```python
from build123d import *

# Parameters (mm, degrees)
PAD_DEPTH       = 5
PAD001_DEPTH    = 30
POCKET_DEPTH    = 162.001
POCKET001_DEPTH = 5
PAD002_DEPTH    = 5
POCKET002_DEPTH = 5.001
SKETCH007_W     = 22.303925
SKETCH007_H     = 15.153027
SKETCH007_W_2   = 15.272888
SKETCH007_H_2   = 13.786167
POCKET003_DEPTH = 3
SKETCH008_W     = 25.606406
SKETCH008_H     = 16.851532
SKETCH008_W_2   = 36.655319
SKETCH008_H_2   = 18.371552
POCKET004_DEPTH = 3
SKETCH009_R     = 1.5
POCKET005_DEPTH = 5
SKETCH010_R     = 3.6
SKETCH010_R_2   = 12.75
POCKET006_DEPTH = 5.001
SKETCH011_W     = 5.6250572961
SKETCH011_H     = 4
POCKET007_DEPTH = 5.001
SKETCH012_R     = 15
POCKET008_DEPTH = 3
SKETCH013_R     = 6.1
POCKET009_DEPTH = 1
SKETCH_R        = 1.4
POCKET010_DEPTH = 3.5
POCKET011_DEPTH = 0.2
SKETCH016_W     = 10
SKETCH016_H     = 12
POCKET013_DEPTH = 2.5
SKETCH018_W     = 7.2
SKETCH018_H     = 7.2
POCKET015_DEPTH = 0.2
POCKET016_DEPTH = 3
CHAMFER_SIZE    = 2.2
CHAMFER001_SIZE = 2.9


with BuildPart() as part:
    # Sketch001 → Pad (new body)
    with BuildSketch(Plane.XY):
        with BuildLine():
            Line((0, 0), (162, 0))
            Line((162, 0), (162, 61))
            ThreePointArc((162, 61), (158.4852813742, 69.4852813742), (150, 73))
            Line((150, 73), (12, 73))
            ThreePointArc((12, 73), (3.5147186258, 69.4852813742), (0, 61))
            Line((0, 61), (0, 0))
        make_face()
    extrude(amount=PAD_DEPTH)

    # Sketch002 (on Face8 of Pad) → Pad001 (join)
    with BuildSketch(Plane.XY.offset(5)):
        Polygon((0, 0), (0, 43), (3, 43), (3, 3), (159, 3), (159, 43), (162, 43), (162, 0), align=None)
    extrude(amount=PAD001_DEPTH)

    # Sketch003 (on Face10 of Pad001) → Pocket (cut, through all)
    with BuildSketch(Plane.YZ.offset(162)):
        Polygon((43, 5), (32.4169947557, 8), (23.0748598999, 18), (3, 27), (3, 35), (43, 35), align=None)
    extrude(amount=-POCKET_DEPTH, mode=Mode.SUBTRACT)

    # Sketch004 (on Face5 of Pocket) → Pocket001 (cut)
    with BuildSketch(Plane.XZ):
        with BuildLine():
            Line((0, 27), (0, 61.0433678259))
            Line((0, 61.0433678259), (162, 61.0433678259))
            Line((162, 61.0433678259), (162, 27))
            ThreePointArc((162, 27), (81, 35), (0, 27))
        make_face()
    extrude(amount=-POCKET001_DEPTH, mode=Mode.SUBTRACT)

    # Sketch005 (on Face7 of Pocket001) → Pad002 (join)
    with BuildSketch(Plane.XY.offset(5)):
        with BuildLine():
            Line((162, 50), (169.5, 50))
            ThreePointArc((172, 47.5), (171.267766953, 49.267766953), (169.5, 50))
            Line((172, 47.5), (172, 40.5))
            ThreePointArc((169.5, 38), (171.267766953, 38.732233047), (172, 40.5))
            Line((169.5, 38), (162, 38))
            Line((162, 38), (162, 50))
        make_face()
        with BuildLine():
            Line((0, 50), (-7.5, 50))
            ThreePointArc((-7.5, 50), (-9.267766953, 49.267766953), (-10, 47.5))
            Line((-10, 47.5), (-10, 40.5))
            ThreePointArc((-10, 40.5), (-9.267766953, 38.732233047), (-7.5, 38))
            Line((-7.5, 38), (0, 38))
            Line((0, 38), (0, 50))
        make_face()
        with BuildLine():
            Line((20.5, 73), (40.5, 73))
            Line((40.5, 73), (40.5, 80))
            ThreePointArc((40.5, 80), (39.6213203436, 82.1213203436), (37.5, 83))
            Line((37.5, 83), (23.5, 83))
            ThreePointArc((23.5, 83), (21.3786796564, 82.1213203436), (20.5, 80))
            Line((20.5, 80), (20.5, 73))
        make_face()
        with BuildLine():
            Line((121.5, 73), (141.5, 73))
            Line((141.5, 73), (141.5, 80))
            ThreePointArc((141.5, 80), (140.6213203436, 82.1213203436), (138.5, 83))
            Line((138.5, 83), (124.5, 83))
            ThreePointArc((124.5, 83), (122.3786796564, 82.1213203436), (121.5, 80))
            Line((121.5, 80), (121.5, 73))
        make_face()
    extrude(amount=-PAD002_DEPTH)

    # Sketch006 (on Face56 of Pad002) → Pocket002 (cut, through all)
    with BuildSketch(Plane.XY.offset(5)):
        with BuildLine():
            ThreePointArc((26, 80.5), (23.5, 78), (26, 75.5))
            Line((26, 75.5), (35, 75.5))
            ThreePointArc((35, 75.5), (37.5, 78), (35, 80.5))
            Line((35, 80.5), (26, 80.5))
        make_face()
        with BuildLine():
            ThreePointArc((127, 80.5), (124.5, 78), (127, 75.5))
            Line((127, 75.5), (136, 75.5))
            ThreePointArc((136, 75.5), (138.5, 78), (136, 80.5))
            Line((136, 80.5), (127, 80.5))
        make_face()
        with BuildLine():
            ThreePointArc((-15.2672618866, 46), (-17.2672618866, 44), (-15.2672618866, 42))
            Line((-15.2672618866, 42), (-6, 42))
            ThreePointArc((-6, 42), (-4, 44), (-6, 46))
            Line((-6, 46), (-15.2672618866, 46))
        make_face()
        with BuildLine():
            ThreePointArc((180.8359560682, 42), (182.8359560682, 44), (180.8359560682, 46))
            Line((180.8359560682, 46), (168, 46))
            ThreePointArc((168, 46), (166, 44), (168, 42))
            Line((168, 42), (180.8359560682, 42))
        make_face()
    extrude(amount=-POCKET002_DEPTH, mode=Mode.SUBTRACT)

    # Sketch007 (on Face29 of Pocket002) → Pocket003 (cut)
    with BuildSketch(Plane.XY.offset(5)):
        with Locations((-11.1519625, 45.5765135)):
            Rectangle(SKETCH007_W, SKETCH007_H)
        with Locations((169.636444, 43.1069165)):
            Rectangle(SKETCH007_W_2, SKETCH007_H_2)
    extrude(amount=-POCKET003_DEPTH, mode=Mode.SUBTRACT)

    # Sketch008 (on Face4 of Pocket003) → Pocket004 (cut)
    with BuildSketch(Plane(origin=(0, 0, 0), x_dir=(1, 0, 0), z_dir=(0, 0, -1))):
        with Locations((27.696797, -81.425766)):
            Rectangle(SKETCH008_W, SKETCH008_H)
        with Locations((139.8276595, -82.185776)):
            Rectangle(SKETCH008_W_2, SKETCH008_H_2)
    extrude(amount=-POCKET004_DEPTH, mode=Mode.SUBTRACT)

    # Sketch009 (on Face29 of Pocket004) → Pocket005 (cut)
    with BuildSketch(Plane.XY.offset(5)):
        with Locations((138.5, 78)):
            Circle(SKETCH009_R)
        with Locations((23.5, 78)):
            Circle(SKETCH009_R)
    extrude(amount=-POCKET005_DEPTH, mode=Mode.SUBTRACT)

    # Sketch010 (on Face65 of Pocket005) → Pocket006 (cut, through all)
    with BuildSketch(Plane.XY.offset(5)):
        with Locations((68.4, 38)):
            Circle(SKETCH010_R)
        with Locations((31.0483132961, 45)):
            Circle(SKETCH010_R_2)
        Polygon((88.4, 55), (151, 55), (151, 16), (138.5, 16), (136.5000000003, 14), (102.9, 14), (100.9, 16), (88.4, 16), align=None)
    extrude(amount=-POCKET006_DEPTH, mode=Mode.SUBTRACT)

    # Sketch011 (on Face69 of Pocket006) → Pocket007 (cut, through all)
    with BuildSketch(Plane.XY.offset(5)):
        with Locations((42.985784648, 45)):
            Rectangle(SKETCH011_W, SKETCH011_H)
    extrude(amount=-POCKET007_DEPTH, mode=Mode.SUBTRACT)

    # Sketch012 (on Face42 of Pocket007) → Pocket008 (cut)
    with BuildSketch(Plane.XY.offset(5)):
        with Locations((31.0483132961, 45)):
            Circle(SKETCH012_R)
    extrude(amount=-POCKET008_DEPTH, mode=Mode.SUBTRACT)

    # Sketch013 (on Face72 of Pocket008) → Pocket009 (cut)
    with BuildSketch(Plane.XY.offset(5)):
        with Locations((68.4, 38)):
            Circle(SKETCH013_R)
    extrude(amount=-POCKET009_DEPTH, mode=Mode.SUBTRACT)

    # Sketch (on Face4 of Pocket009) → Pocket010 (cut)
    with BuildSketch(Plane(origin=(0, 0, 0), x_dir=(1, 0, 0), z_dir=(0, 0, -1))):
        with Locations((85.9, -16)):
            Circle(SKETCH_R)
        with Locations((153.5, -16)):
            Circle(SKETCH_R)
        with Locations((85.9, -55)):
            Circle(SKETCH_R)
        with Locations((153.5, -55)):
            Circle(SKETCH_R)
    extrude(amount=-POCKET010_DEPTH, mode=Mode.SUBTRACT)

    # Sketch014 (on Face81 of Pocket010) → Pocket011 (cut)
    with BuildSketch(Plane(origin=(0, 0, 3.5), x_dir=(1, 0, 0), z_dir=(0, 0, -1))):
        with BuildLine():
            Line((85.15, -56.1821590418), (85.15, -53.8178409582))
            ThreePointArc((86.65, -53.8178409582), (85.9, -53.6310250587), (85.15, -53.8178409582))
            Line((86.65, -56.1821590418), (86.65, -53.8178409582))
            ThreePointArc((85.15, -56.1821590418), (85.9, -56.3158445643), (86.65, -56.1821590418))
        make_face()
        with BuildLine():
            Line((152.75, -17.1821590418), (152.75, -14.8178409582))
            ThreePointArc((154.25, -14.8178409582), (153.5, -14.6), (152.75, -14.8178409582))
            Line((154.25, -14.8178409582), (154.25, -17.1821590418))
            ThreePointArc((152.75, -17.1821590418), (153.5, -17.4), (154.25, -17.1821590418))
        make_face()
        with BuildLine():
            Line((152.75, -56.1821590418), (152.75, -53.8178409582))
            ThreePointArc((154.25, -53.8178409582), (153.5, -53.6), (152.75, -53.8178409582))
            Line((154.25, -56.1821590418), (154.25, -53.8178409582))
            ThreePointArc((152.75, -56.1821590418), (153.5, -56.4), (154.25, -56.1821590418))
        make_face()
        with BuildLine():
            Line((85.15, -17.1821590418), (85.15, -14.8178409582))
            ThreePointArc((86.65, -14.8178409582), (85.9, -14.6), (85.15, -14.8178409582))
            Line((86.65, -14.8178409582), (86.65, -17.1821590418))
            ThreePointArc((85.15, -17.1821590418), (85.9, -17.4337278664), (86.65, -17.1821590418))
        make_face()
    extrude(amount=-POCKET011_DEPTH, mode=Mode.SUBTRACT)

    # Sketch016 → Pocket013 (cut)
    with BuildSketch(Plane(origin=(0, 0, 0), x_dir=(1, 0, 0), z_dir=(0, 0, -1))):
        with Locations((68.4, -37)):
            Rectangle(SKETCH016_W, SKETCH016_H)
    extrude(amount=-POCKET013_DEPTH, mode=Mode.SUBTRACT)

    # Sketch018 → Pocket015 (cut)
    with BuildSketch(Plane.XZ.offset(-55.75)):
        with Locations((68.4, -38)):
            Rectangle(SKETCH018_W, SKETCH018_H)
    extrude(amount=-POCKET015_DEPTH, mode=Mode.SUBTRACT)

    # Sketch019 (on Face4 of Pocket015) → Pocket016 (cut)
    with BuildSketch(Plane(origin=(0, 0, 0), x_dir=(1, 0, 0), z_dir=(0, 0, -1))):
        with BuildLine():
            ThreePointArc((88, -25), (86.5, -23.5), (85, -25))
            Line((85, -25), (85, -45))
            ThreePointArc((85, -45), (86.5, -46.5), (88, -45))
            Line((88, -45), (88, -25))
        make_face()
    extrude(amount=-POCKET016_DEPTH, mode=Mode.SUBTRACT)

    # Chamfer
    chamfer_edges = [part.edges().sort_by_distance(p)[0] for p in [
        (88.4, 29.5, 5),
        (119.7, 55, 5),
        (151, 49, 5),
        (151, 29.5, 5),
        (144.75, 16, 5),
        (137.5, 15, 5),
        (119.7, 14, 5),
        (101.9, 15, 5),
        (94.65, 16, 5),
    ]]
    chamfer(chamfer_edges, length=CHAMFER_SIZE)

    # Chamfer001
    chamfer001_edges = [part.edges().sort_by_distance(p)[0] for p in [
        (30.046074, 59.96648, 5),
    ]]
    chamfer(chamfer001_edges, length=CHAMFER001_SIZE)


solid = part.part
```
The model under review builds one solid part; all positions refer to its coordinate system, in mm. A direction names the side the tool comes from. Round coordinates to 2 decimals unless told otherwise and drop trailing zeros. Loops run counter-clockwise (first coordinate to the right, second up) from the corner with the lowest first, then second, coordinate; pieces in that order, holes last.
1) Consider section D-D on z = 31.5. State the section outline as (x, y) points, then the cut area to 3 significant figures.
Values follow:
outline: (27.28, 0) - (134.72, 0) - (134.72, 3) - (27.28, 3) - close
area: 322 mm2
2) The part is to be moulded in two halves that separate along Y. For faces 1 (the face through (82, 0, 17)), 2 (the face through (68, 34, 2.5)), 3 (the face through (131, 75, 3)), 4 (the face through (160.521, 13.178, 22.437)), say which applies: pulls with the +Y half, pulls with the -Y half, needs draft (parallel to the pull), parting line crosses it, or undercut.
Values follow:
face 1: pulls with the -Y half
face 2: undercut
face 3: needs draft
face 4: pulls with the +Y half
3) Consider section C-C on y = 71. State the section outline as (x, z) points, then the cut area to 3 significant figures.
Values follow:
outline: (5.37, 0) - (156.63, 0) - (156.63, 5) - (5.37, 5) - close
area: 756 mm2
4) Clearance check with flat-ended pins moving along their axes: P1, Ø12, axis at y = 17, z = 8, coming from the +X side; P2, Ø2, axis at x = 170, z = 1.5, coming from the +Y side; P3, Ø0.8, axis at x = 86, y = 55, coming from the -Z side; P4, Ø8, axis at x = 142, y = 21.5, coming from the +Z side. State where each tip first meets the part, or that it passes through.
Values follow:
P1: stops at x = 162
P2: stops at y = 50
P3: stops at z = 3.7
P4: passes through
5) Consider section A-A on x = 94. State the section outline as (y, z) points, then the cut area to 3 significant figures.
Values follow:
outline: (0, 0) - (16, 0) - (16, 2.8) - (13.8, 5) - (3, 5) - (3, 34.8) - (0, 34.8) - close; (55, 0) - (73, 0) - (73, 5) - (57.2, 5) - (55, 2.8) - close
area: 255 mm2
6) Consider section B-B on z = 10.5. State the section outline as (x, y) points, then the cut area to 3 significant figures.
Values follow:
outline: (0, 0) - (162, 0) - (162, 30.08) - (159, 30.08) - (159, 3) - (3, 3) - (3, 30.08) - (0, 30.08) - close
area: 648 mm2
7) Tool access review of faces 5 (the face through (3, 14, 13)), 6 (the face through (165.8, 44.1, 2)), 7 (the face through (82, 73, 2)), 8 (the face through (63.9, 42.12, 4.51)): name each direction out of +Z, -Z, +X, -X, +Y, -Y from which nothing blocks a thin tool from reaching the whole face with its end or side.
Values follow:
face 5: +Z, +Y
face 6: +Z, +X, +Y, -Y
face 7: -Z, +Y
face 8: +Z
8) Wall thickness on line 1 along Y through (x, z) = (68, 3); line 2 along X through (y, z) = (17.5, 20); line 3 along Y through (x, z) = (23.5, 4.05): over which ranges is each line inside the solid? List them lowest first.
Values follow:
line 1: y = 0 to 34.42, 41.58 to 73
line 2: x = 0 to 3, 159 to 162
line 3: y = 0 to 29.82, 60.18 to 76.5, 79.5 to 83
